Design review of the part built by this model. Coordinates are the model's own, in mm. A direction names the side the tool comes from. Give positions to 0.01 mm unless a question says otherwise; leave off trailing zeros. Write each loop counter-clockwise with the first axis right and the second up, starting at its lowest first coordinate (ties: lowest second). Pieces come first, ordered by that corner, then holes. Notation, with made-up numbers: (14.5, -37) -> (51.5, -37) arc R25 cw to (51.5, -1) -> close; hole circle Ø3 at (56.5, 36.25). An arc over 180 degrees is marked (long way). Write each question's results on one line, items separated by ' | '. Start each with the question number.
(1) Take a section at B-B (z = 16.5). State the section outline as (x, y) points, plus the area to 3 significant figures.
(2) To check wall thickness, follow probe 1 along X at (y, z) = (1.25, 15); probe 2 along X at (y, z) = (-8.75, 11.5); probe 3 along X at (y, z) = (-18.25, 10). State the ranges of each line that lie inside material, in increasing order.
(3) Clearance check with flat-ended pins moving along their axes: pin 1 (2.5 mm diameter, centred on y = 0.5, z = 10.5, fed in from +X); pin 2 (3 mm diameter, centred on x = -1.5, z = 10.5, fed in from +Y); pin 3 (10 mm diameter, centred on y = -10.5, z = 15, fed in from -X). State where each tip first meets the part, or that it passes through.
(4) Take a section at A-A (y = -18). State the section outline as (x, z) points.
(5) For faces 1 (the face through (-16, -10, 6.35)), 2 (the face through (-8, -23.063, 9)), 3 (the face through (-5.61, 0, 13)), 4 (the face through (27, -10, 6.35)), 5 (the face through (31.075, -7, 3)), list the 3-axis set-ups (+Z, -Z, +X, -X, +Y, -Y) from which the entire face can be reached by the end or side of a thin tool; tool diameter is ignored.
(6) Take a section at C-C (x = -5). State the section outline as (y, z) points, plus the area to 3 significant figures.
(7) Mouldability with a two-part tool opening along X and no side actions: class faces 6 (the face through (20, -23.063, 9)), 7 (the face through (23.455, -11, 13)), 8 (the face through (17.105, 0, 13)) as released by +X, released by -X, zero draft, split by the parting line, or undercut.
(8) Take a section at D-D (y = -12.25). State the section outline as (x, z) points, plus the area to 3 significant figures.
from build123d import *

# Parameters (mm, degrees)
F0_W     = 50.8
F0_H     = 25.4
F1_DEPTH = 6.35
F2_R     = 7.62
F3_W     = 35.415467
F3_H     = 25.4
F4_DEPTH = 12.7
F6_DEPTH = 19.051
F7_W     = 22.715467
F7_H     = 5.149726
F8_DEPTH = 12.7


with BuildPart() as f1:
    # F0 (on Top) → F1 (new body)
    with BuildSketch(Plane.XY):
        with Locations((5.675177, -10.363199)):
            Rectangle(F0_W, F0_H)
    extrude(amount=F1_DEPTH)

    # F2
    f2_edges = [f1.edges().sort_by_distance(p)[0] for p in [
        (-19.724823, -23.063199, 3.175),
        (31.075177, -23.063199, 3.175),
    ]]
    fillet(f2_edges, radius=F2_R)

    # F3 (on face) → F4 (join)
    with BuildSketch(Plane.XY.offset(6.35)):
        with Locations((5.747444, -10.363199)):
            Rectangle(F3_W, F3_H)
    extrude(amount=F4_DEPTH)

    # F5 (on face) → F6 (cut, through all)
    with BuildSketch(Plane.XY.offset(19.05)):
        with BuildLine():
            Line((-4.34029, -23.063199), (15.835177, -23.063199))
            ThreePointArc((15.835177, -23.063199), (5.747443, -12.972925), (-4.34029, -23.063199))
        make_face()
    extrude(amount=-F6_DEPTH, mode=Mode.SUBTRACT)

    # F7 (on face) → F8 (cut)
    with BuildSketch(Plane.XY.offset(19.05)):
        with Locations((5.747443, -0.238062)):
            Rectangle(F7_W, F7_H)
    extrude(amount=-F8_DEPTH, mode=Mode.SUBTRACT)


solid = f1.part
Report:
1) outline: (-11.96, -23.06) -> (-4.34, -23.06) arc R10.09 cw to (15.84, -23.06) -> (23.46, -23.06) -> (23.46, 2.34) -> (17.11, 2.34) -> (17.11, -2.81) -> (-5.61, -2.81) -> (-5.61, 2.34) -> (-11.96, 2.34) -> close | area: 623 mm2
2) probe 1: -11.96 to -5.61, 17.11 to 23.46 | probe 2: -11.96 to 23.46 | probe 3: -11.96 to -3.12, 14.61 to 23.46
3) pin 1: x = 23.46 | pin 2: y = -2.81 | pin 3: x = -11.96
4) outline: (-19.28, 0) -> (-2.98, 0) -> (-2.98, 19.05) -> (-11.96, 19.05) -> (-11.96, 6.35) -> (-19.28, 6.35) -> close; (14.47, 0) -> (30.63, 0) -> (30.63, 6.35) -> (23.46, 6.35) -> (23.46, 19.05) -> (14.47, 19.05) -> close
5) face 1: +Z, -X, +Y, -Y | face 2: +Z, -Z, +X, -X, -Y | face 3: +Z, +Y | face 4: +Z, +X, +Y, -Y | face 5: +Z, -Z, +X, +Y, -Y
6) outline: (-23.06, 0) -> (2.34, 0) -> (2.34, 6.35) -> (-2.81, 6.35) -> (-2.81, 19.05) -> (-23.06, 19.05) -> close | area: 418 mm2
7) face 6: zero draft | face 7: released by +X | face 8: undercut
8) outline: (-19.72, 0) -> (31.08, 0) -> (31.08, 6.35) -> (23.46, 6.35) -> (23.46, 19.05) -> (-11.96, 19.05) -> (-11.96, 6.35) -> (-19.72, 6.35) -> close | area: 772 mm2
